from build123d import *

# Parameters (mm, degrees)
F0_W      = 101.6
F0_H      = 42.112397
F1_DEPTH  = 101.6
F2_W      = 50.8
F2_H      = 76.2
F3_DEPTH  = 203.2
F4_W      = 101.6
F4_H      = 20.007362
F5_DEPTH  = 25.4
F6_W      = 101.6
F6_H      = 38.950141
F7_DEPTH  = 50.8
F9_DEPTH  = 101.6
F11_DEPTH = 101.6


with BuildPart() as f1:
    # F0 (on Front) → F1 (new body)
    with BuildSketch(Plane.XZ):
        Polygon((-50.799996, 59.025088), (-101.599996, 59.025088), (-101.599996, -42.574912), (101.600004, -42.574912), (101.600004, 59.025088), (50.800004, 59.025088), (50.800004, 16.912691), (-50.799996, 16.912691), align=None)
        with Locations((4e-06, 37.968889)):
            Rectangle(F0_W, F0_H)
    extrude(amount=F1_DEPTH)

    # F2 (on face) → F3 (cut)
    with BuildSketch(Plane.YZ.offset(101.600004)):
        with Locations((-76.2, 20.925088)):
            Rectangle(F2_W, F2_H)
    extrude(amount=-F3_DEPTH, mode=Mode.SUBTRACT)

    # F4 (on face) → F5 (cut)
    with BuildSketch(Plane.XY.offset(-17.174912)):
        with Locations((4e-06, -91.596319)):
            Rectangle(F4_W, F4_H)
    extrude(amount=-F5_DEPTH, mode=Mode.SUBTRACT)

    # F6 (on face) → F7 (cut)
    with BuildSketch(Plane.XZ.offset(50.8)):
        with Locations((4e-06, 39.550017)):
            Rectangle(F6_W, F6_H)
    extrude(amount=-F7_DEPTH, mode=Mode.SUBTRACT)

    # F8 (on face) → F9 (cut)
    with BuildSketch(Plane.XZ.offset(50.8)):
        Polygon((-76.199996, 59.025088), (-101.599996, 59.025088), (-101.599996, 33.625088), align=None)
    extrude(amount=-F9_DEPTH, mode=Mode.SUBTRACT)

    # F10 (on face) → F11 (cut)
    with BuildSketch(Plane.XZ.offset(50.8)):
        Polygon((76.200004, 59.025088), (101.600004, 33.625088), (101.600004, 59.025088), align=None)
    extrude(amount=-F11_DEPTH, mode=Mode.SUBTRACT)


solid = f1.part
Geometry check sheet. Reference: the model listing, model coordinates, mm. A direction names the side the tool comes from. Give positions to 0.01 mm unless a question says otherwise; leave off trailing zeros. Order: outer loops, then holes, each group sorted by start corner. A loop starts at its lowest first (then second) coordinate and runs counter-clockwise, first axis right, second up.
1. Sectioned sample at C-C (y = -31). Record the boundary of the cut face in (x, z), then the cut area to 3 significant figures.
Completed:
outline: (-101.6, -42.57) - (101.6, -42.57) - (101.6, 33.63) - (76.2, 59.03) - (50.8, 59.03) - (50.8, 20.07) - (-50.8, 20.07) - (-50.8, 59.03) - (-76.2, 59.03) - (-101.6, 33.63) - close
area: 16,000 mm2
2. Sectioned sample at A-A (y = -89). Record the boundary of the cut face in (x, z), then the cut area to 3 significant figures.
Completed:
outline: (-101.6, -42.57) - (-50.8, -42.57) - (-50.8, -17.17) - (-101.6, -17.17) - close; (50.8, -42.57) - (101.6, -42.57) - (101.6, -17.17) - (50.8, -17.17) - close
area: 2,580 mm2
3. Draft check along X on faces 6 (the face through (101.6, -39, -13)), 7 (the face through (-1, -26, 20.075)), 8 (the face through (-63, -25, 59.025)), 9 (the face through (-1, -81.593, -30)). Enter one of: pulls with the +X half, pulls with the -X half, needs draft (parallel to the pull), parting line crosses it, or undercut.
Completed:
face 6: pulls with the +X half
face 7: undercut
face 8: needs draft
face 9: undercut
4. Depth check by flat-ended pin: pin 1 (20.5 mm diameter, centred on x = -13, z = -31.5, fed in from -Y); pin 2 (19.5 mm diameter, centred on y = -27, z = 37.5, fed in from +X); pin 3 (5 mm diameter, centred on x = 67.5, y = -74.5, fed in from +Z); pin 4 (19.5 mm diameter, centred on y = -18, z = 45, fed in from -X). Enter the tip coordinate at first touch or a pass-through.
Completed:
pin 1: stops at y = -81.59
pin 2: stops at x = 101.6
pin 3: stops at z = -17.17
pin 4: stops at x = -99.98
5. Access from +Z, -Z, +X, -X, +Y, -Y to the whole of each face (thin tool, end or side, straight path). Record for faces 1 (the face through (-1, -50, -42.575)), 2 (the face through (50.8, -92, -30)), 3 (the face through (1, -50.8, 12)), 4 (the face through (76, -101.6, -30)), 5 (the face through (50.8, -26, 39)).
Completed:
face 1: -Z, +X, -X, +Y, -Y
face 2: +Z, -Z, -Y
face 3: +Z, +X, -X, -Y
face 4: +Z, -Z, +X, -X, -Y
face 5: +Z, +Y, -Y
6. Sectioned sample at D-D (x = -18). Record the boundary of the cut face in (y, z).
Completed:
outline: (-81.59, -42.57) - (0, -42.57) - (0, 20.07) - (-50.8, 20.07) - (-50.8, -17.17) - (-81.59, -17.17) - close
7. Scan lines: line 1 (X direction, y = -96.5, z = -29); line 2 (Y direction, x = 46, z = -13.5); line 3 (Z direction, x = -4, y = -73). Record each from-to range of solid material in increasing order.
Completed:
line 1: x = -101.6 to -50.8, 50.8 to 101.6
line 2: y = -50.8 to 0
line 3: z = -42.57 to -17.17
8. Sectioned sample at B-B (z = 27). Record the boundary of the cut face in (x, y).
Completed:
outline: (-101.6, -50.8) - (-50.8, -50.8) - (-50.8, 0) - (-101.6, 0) - close; (50.8, -50.8) - (101.6, -50.8) - (101.6, 0) - (50.8, 0) - close
